Read the model definition and answer for the solid it produces. Units are mm, in the model's axes. Give positions to 0.01 mm unless a question says otherwise; leave off trailing zeros. Order: outer loops, then holes, each group sorted by start corner. A loop starts at its lowest first (then second) coordinate and runs counter-clockwise, first axis right, second up. Notation, with made-up numbers: (40, 7.5) - (94, 7.5) arc R20 cw to (94, 42.5) - close; hole circle Ø2 at (-34.75, 42). An arc over 180 degrees is marked (long way). Return JSON: item names as keys, results as strings.
```python
from build123d import *

# Parameters (mm, degrees)
SKETCH027_R           = 71
SKETCH028_R           = 58
SKETCH025_R           = 75
SKETCH026_R           = 60
POCKET005_DEPTH       = 31
POLARPATTERN007_COUNT = 4


with BuildPart() as loft001:
    # Sketch027 → Loft001 section 0
    with BuildSketch(Plane.XY.offset(10)):
        Circle(SKETCH027_R)
    # Sketch028 → Loft001 section 1
    with BuildSketch(Plane.XY.offset(50)):
        Circle(SKETCH028_R)
    loft()


with BuildPart() as support:
    # Sketch025 → Loft section 0
    with BuildSketch(Plane.XY.offset(10)):
        Circle(SKETCH025_R)
    # Sketch026 → Loft section 1
    with BuildSketch(Plane.XY.offset(50)):
        Circle(SKETCH026_R)
    loft()

    # Cut: cut Loft001
    add(loft001.part, mode=Mode.SUBTRACT)

    # Sketch029 → Pocket005 (cut)
    with BuildSketch(Plane(origin=(-60, -60, 0), x_dir=(-0.707107, 0.707107, 0), z_dir=(0.707107, 0.707107, 0))):
        Polygon((9.467248, 65.201898), (0, 19.378601), (-9.467248, 65.201898), align=None)
    pocket005 = extrude(amount=POCKET005_DEPTH, mode=Mode.SUBTRACT)

    # PolarPattern007: Pocket005 ×4 about axis
    polarpattern007_axis = Axis((0, 0, 0), (0, 0, 1))
    for i in range(1, POLARPATTERN007_COUNT):
        add(pocket005.rotate(polarpattern007_axis, i * 360 / POLARPATTERN007_COUNT), mode=Mode.SUBTRACT)


solid = support.part
```
Q1. Determine the mould class of faces 1 (the flat face through (43.96, -48.123, 33.627)), 2 (the flat face through (-59, 0, 50)), 3 (the conical face through (28.022, -53.876, 48.058)) for opening direction Y: released by +Y, released by -Y, zero draft, split by the parting line, or undercut.
Values:
{"face 1": "undercut", "face 2": "zero draft", "face 3": "split by the parting line"}
Q2. Consider L1, parallel to X at y = 43, z = 14.5; L2, parallel to Y at x = -41, z = 30.5; L3, parallel to Y at x = 1.5, z = 46. Determine where each line is inside the solid, lowest interval first.
Values:
{"L1": "x = -59.38 to -54.65, 54.65 to 59.38", "L2": "y = -53.39 to -49.58, 49.58 to 53.39", "L3": "y = -61.48 to -59.28, 59.28 to 61.48"}
Q3. Given pin 1 (1 mm diameter, centred on y = -0.5, z = 25.5, fed in from -X); pin 2 (10 mm diameter, centred on x = -15.5, z = 34, fed in from -Y); pin 3 (6 mm diameter, centred on y = 2.5, z = 19, fed in from +X), each flat-ended and moving along its own axis, determine where each tip first touches the part or whether it passes through.
Values:
{"pin 1": "stops at x = -69.37", "pin 2": "stops at y = -66.36", "pin 3": "stops at x = 72.71"}
Q4. A cutting plane is placed at B-B (z = 22.5). Write down the section's boundary in (x, y) (1 decimal), and give its area (3 significant figures).
Values:
{"outline": "(-50.2, -49.3) - (-47.8, -46.9) arc R66.9 cw to (-47.8, 46.9) - (-50.2, 49.3) arc R70.3 ccw to start; (-49.3, -50.2) arc R70.3 ccw to (49.3, -50.2) - (46.9, -47.8) arc R66.9 cw to (-46.9, -47.8) - close; (-49.3, 50.2) - (-46.9, 47.8) arc R66.9 cw to (46.9, 47.8) - (49.3, 50.2) arc R70.3 ccw to start; (47.8, -46.9) - (50.2, -49.3) arc R70.3 ccw to (50.2, 49.3) - (47.8, 46.9) arc R66.9 cw to start", "area": "1,440 mm²"}
Q5. A cutting plane is placed at A-A (x = 0). Write down the section's boundary in (y, z).
Values:
{"outline": "(-75, 10) - (-71, 10) - (-58, 50) - (-60, 50) - close; (58, 50) - (71, 10) - (75, 10) - (60, 50) - close"}
Q6. A cutting plane is placed at C-C (z = 32.5). Write down the section's boundary in (x, y) (1 decimal).
Values:
{"outline": "(-48.9, -45.1) - (-46.9, -43.1) arc R63.7 cw to (-46.9, 43.1) - (-48.9, 45.1) arc R66.6 ccw to start; (-45.1, -48.9) arc R66.6 ccw to (45.1, -48.9) - (43.1, -46.9) arc R63.7 cw to (-43.1, -46.9) - close; (-45.1, 48.9) - (-43.1, 46.9) arc R63.7 cw to (43.1, 46.9) - (45.1, 48.9) arc R66.6 ccw to start; (46.9, -43.1) - (48.9, -45.1) arc R66.6 ccw to (48.9, 45.1) - (46.9, 43.1) arc R63.7 cw to start"}
